Autodesk Inventor part; units mm, degrees
ref_plane "Work Plane1" through (0, 10.287, 0) normal (0, 1, 0) x (-1, 0, 0)
ref_plane "YZ Plane" through (0, 0, 0) normal (1, 0, 0) x (0, 1, 0)
ref_plane "XY Plane" through (0, 0, 0) normal (0, 0, 1) x (1, 0, 0)
sketch "Sketch1" plane through (0, 0, 0) normal (0, 0, 1) x (1, 0, 0)
  circle A0 centre (0, 0) radius 10.287
  dimension "d0" = 20.574
extrude "Extrusion1" add sketch "Sketch1" along normal blind 254
ref_plane "Work Plane1" through (0, 10.287, 0) normal (0, 1, 0) x (-1, 0, 0)
sketch "Sketch2" plane through (0, 10.287, 0) normal (0, 1, 0) x (-1, 0, 0)
  line L0 (5.715, 241.8104) -> (0, 238.5109)
  line L1 (0, 238.5109) -> (-5.715, 241.8104)
  line L2 (-5.715, 241.8104) -> (-5.715, 248.4096)
  line L3 (-5.715, 248.4096) -> (0, 251.7091)
  line L4 (0, 251.7091) -> (5.715, 248.4096)
  line L5 (5.715, 248.4096) -> (5.715, 241.8104)
  line L6 (5.715, 5.5904) -> (0, 2.2909)
  line L7 (0, 2.2909) -> (-5.715, 5.5904)
  line L8 (-5.715, 5.5904) -> (-5.715, 12.1896)
  line L9 (-5.715, 12.1896) -> (0, 15.4891)
  line L10 (0, 15.4891) -> (5.715, 12.1896)
  line L11 (5.715, 12.1896) -> (5.715, 5.5904)
  line L12 (10.287, 0) -> (10.287, 254)
  line L13 (10.287, 254) -> (-10.287, 254)
  line L14 (-10.287, 0) -> (10.287, 0)
  point P0 (0, 0)
  point P1 (0, 245.11)
  point P2 (0, 8.89)
  dimension "d3" = 11.43
  dimension "d4" = 11.43
  dimension "d5" = 8.89
  dimension "d6" = 8.89
  dimension "d7" = 10.287
  dimension "d8" = 10.287
extrude "Extrusion2" add sketch "Sketch2" along normal mid plane 12.7
sketch "Sketch3" plane through (0, 16.637, 0) normal (0, 1, 0) x (1, 0, 0)
  line L0 (0, -2.2909) -> (-5.715, -5.5904)
  line L1 (-5.715, -5.5904) -> (-5.715, -12.1896)
  line L2 (-5.715, -12.1896) -> (0, -15.4891)
  line L3 (0, -15.4891) -> (5.715, -12.1896)
  line L4 (5.715, -12.1896) -> (5.715, -5.5904)
  line L5 (5.715, -5.5904) -> (0, -2.2909)
  line L6 (0, -238.5109) -> (-5.715, -241.8104)
  line L7 (-5.715, -241.8104) -> (-5.715, -248.4096)
  line L8 (-5.715, -248.4096) -> (0, -251.7091)
  line L9 (0, -251.7091) -> (5.715, -248.4096)
  line L10 (5.715, -248.4096) -> (5.715, -241.8104)
  line L11 (5.715, -241.8104) -> (0, -238.5109)
  circle A0 centre (0, -245.1051) radius 5.08
  circle A1 centre (0, -8.8949) radius 5.08
  point P0 (0, 0)
  dimension "d11" = 10.16
  dimension "d12" = 10.16
  dimension "d13" = 5.715
  dimension "d14" = 5.715
  dimension "d15" = 6.604
  dimension "d16" = 6.604
extrude "Extrusion3" add sketch "Sketch3" along normal blind 2.1209 contours A0 | A1
sketch "Sketch6" plane through (0, 0, 0) normal (0, 0, -1) x (-1, 0, 0)
  circle A0 centre (0, 0) radius 10.287
  circle A1 centre (0, 0) radius 7.9375
  dimension "d33" = 15.875
extrude "Extrusion5" add sketch "Sketch6" along normal blind 0.254 contours A1
sketch "Sketch7" plane through (0, 0, -0.254) normal (0, 0, -1) x (-1, 0, 0)
  circle A0 centre (0, 0) radius 7.9375
  line L0 (0, 16.637) -> (5.715, 16.637)
  line L1 (-6.5762, 4.445) -> (6.5762, 4.445)
  line L2 (-6.5762, -4.445) -> (6.5762, -4.445)
  arc A1 (-6.5762, 4.445) -> (-6.5762, -4.445) centre (0, 0) ccw
  arc A2 (6.5762, -4.445) -> (6.5762, 4.445) centre (0, 0) ccw
  dimension "d42" = 0
  dimension "d44" = 8.89
  dimension "d45" = 4.445
thread "Thread1"
extrude "Extrusion7" add sketch "Sketch7" along normal blind 15.621 contours A0 L2 L1
sketch "Sketch8" plane through (-6.5762, 4.445, -0.254) normal (0, 1, 0) x (1, 0, 0)
  circle A0 centre (6.5737, 9.271) radius 3.175
  line L0 (13.1523, 0) -> (13.1523, 15.621)
  line L1 (0, 15.621) -> (13.1523, 15.621)
  point P0 (6.5762, -0.254)
  dimension "d48" = 6.35
  dimension "d49" = 6.5786
  dimension "d50" = 6.35
extrude "Extrusion8" cut sketch "Sketch8" against normal blind 15.621
sketch "Sketch9" plane through (0, 0, 254) normal (0, 0, 1) x (1, 0, 0)
  circle A0 centre (0, 0) radius 7.9375
  circle A1 centre (0, 0) radius 7.9375
  dimension "d53" = 15.875
extrude "Extrusion9" add sketch "Sketch9" along normal blind 2.54
sketch "Sketch10" plane through (0, 0, 254) normal (0, 0, 1) x (1, 0, 0)
  circle A0 centre (0, 0) radius 7.9375
  circle A1 centre (0, 0) radius 10.287
  line L0 (-9.652, 3.5583) -> (-9.652, -3.5583)
  line L1 (9.652, 3.5583) -> (9.652, -3.5583)
  line L2 (-5.715, 16.637) -> (-5.715, 8.5534)
  arc A2 (9.652, -3.5583) -> (9.652, 3.5583) centre (0, 0) ccw
  arc A3 (-9.652, 3.5583) -> (-9.652, -3.5583) centre (0, 0) ccw
  dimension "d58" = 19.304
  dimension "d59" = 9.652
extrude "Extrusion10" cut sketch "Sketch10" against normal blind 12.7 contours A1 L1 | A1 L0
sketch "Sketch11" plane through (0, 0, 256.54) normal (0, 0, 1) x (1, 0, 0)
  circle A0 centre (0, 0) radius 6.985
  dimension "d62" = 13.97
extrude "Extrusion11" add sketch "Sketch11" along normal blind 10.795
thread "Thread2"
sketch "Sketch12" plane through (0, 0, 267.335) normal (0, 0, 1) x (1, 0, 0)
  circle A0 centre (0, 0) radius 1.5875
  dimension "d67" = 3.175
extrude "Extrusion12" cut sketch "Sketch12" against normal blind 187.96
equation "\"d4\" = d3"
equation "\"d14\" = d13"
equation "\"d15\" = d16"
properties part number "RobotArm Cylinder"
Here's how the part is built. I have some questions about the finished solid (model axes, mm). A direction names the side the tool comes from. Round coordinates to 2 decimals unless told otherwise and drop trailing zeros. Order: outer loops, then holes, each group sorted by start corner. A loop starts at its lowest first (then second) coordinate and runs counter-clockwise, first axis right, second up. Notation, with made-up numbers: M 29.25,-26.5 L 69.25,-26.5 A18 ccw 69.25,0.5 Z; hole C 36,36.25 d2. An arc over 180 degrees is marked long. Answer in a Markdown table with one row per item.
Item 1: I'm going to push flat-ended pins straight in: pin 1 (4 mm diameter, centred on x = -1, y = -7, fed in from -Z); pin 2 (1 mm diameter, centred on x = -7, y = -5.5, fed in from -Z); pin 3 (5.5 mm diameter, centred on y = 14, z = 246.5, fed in from +X) (3 decimals). Where does each tip first touch, or does it pass through?
A:
| item | result |
|---|---|
| pin 1 | stops at z = -0.25 |
| pin 2 | stops at z = 0 |
| pin 3 | stops at x = 5.715 |
Item 2: Imagine slicing it at A-A, the plane z = 133. Write out the boundary of the cut face in (x, y) (1 decimal), and give its area (3 significant figures).
A:
| item | result |
|---|---|
| outline | C 0,0 d20.6; hole C 0,0 d3.2 |
| area | 325 mm2 |
Item 3: Thinking about a two-plate mould opening in Z: for faces 6 (the face through (-1.101, 17.683, 240.146)), 7 (the face through (0, -4.445, -6)), 8 (the face through (0, 0, -15.875)), which applies, +Z half, -Z half, draft (parallel to the pull), parting line (faces both ways), or undercut?
A:
| item | result |
|---|---|
| face 6 | undercut |
| face 7 | draft |
| face 8 | -Z half |
Item 4: If I drill on L1, parallel to Y at x = 0, z = 167; L2, parallel to Y at x = 6.5, z = 169; L3, parallel to Z at x = -5, y = -7.5, over which ranges is the centre line in solid material (lowest first)? Write a range as from..to.
A:
| item | result |
|---|---|
| L1 | y = -10.29..-1.59, 1.59..10.29 |
| L2 | y = -7.97..7.97 |
| L3 | z = 0..254 |
Item 5: Imagine slicing it at B-B, the plane z = 29.5. Write out the boundary of the cut face in (x, y), and give its area (3 significant figures).
A:
| item | result |
|---|---|
| outline | C 0,0 d20.57 |
| area | 332 mm2 |
Item 6: For faces 1 (the face through (-2.898, 13.437, 240.184)), 2 (the face through (2.82, 13.44, 3.92)), 3 (the face through (5.715, 13, 245)), 4 (the face through (2.898, 13.437, 13.816)), 5 (the face through (-0.909, -6.926, 261.862)), which set-ups out of +Z, -Z, +X, -X, +Y, -Y let a thin tool reach every point of the face, with its end or its side?
A:
| item | result |
|---|---|
| face 1 | -X, +Y |
| face 2 | -Z, +X, +Y |
| face 3 | +Z, -Z, +X, +Y |
| face 4 | +X, +Y |
| face 5 | +Z |
